Verification items for the finished model (mm, model axes). A direction names the side the tool comes from. Give positions to 0.01 mm unless a question says otherwise; leave off trailing zeros. Write each loop counter-clockwise with the first axis right and the second up, starting at its lowest first coordinate (ties: lowest second). Pieces come first, ordered by that corner, then holes. Notation, with made-up numbers: (67.5, 51.5) -> (124.5, 51.5) arc R11 ccw to (124.5, 56.5) -> close; hole circle Ø10 at (37.25, 61). An arc over 180 degrees is marked (long way). Answer as CSV lines item,"result".
Autodesk Inventor part; units mm, degrees
ref_plane "YZ Plane" through (0, 0, 0) normal (1, 0, 0) x (0, 1, 0)
ref_plane "XZ Plane" through (0, 0, 0) normal (0, 1, 0) x (-1, 0, 0)
ref_plane "XY Plane" through (0, 0, 0) normal (0, 0, 1) x (1, 0, 0)
sketch "Sketch1" plane through (0, 0, 0) normal (0, 1, 0) x (-1, 0, 0)
  circle A0 centre (-31.5089, -30.9076) radius 2.1844
  circle A1 centre (-31.5089, 40.6188) radius 2.1844
  circle A2 centre (44.6911, -30.9076) radius 2.1844
  circle A3 centre (44.6911, 40.6188) radius 2.1844
  circle A4 centre (44.6911, 40.6188) radius 6.35
  circle A5 centre (44.6911, -30.9076) radius 6.35
  circle A6 centre (-31.5089, -30.9076) radius 6.35
  circle A7 centre (-31.5089, 40.6188) radius 6.35
  line L0 (44.6911, 46.9688) -> (-31.5089, 46.9688)
  line L1 (-37.8589, 40.6188) -> (-37.8589, -30.9076)
  line L2 (-31.5089, -37.2576) -> (44.6911, -37.2576)
  line L3 (51.0411, -30.9076) -> (51.0411, 40.6188)
  line L4 (44.6911, 34.2688) -> (-31.5089, 34.2688)
  line L5 (-25.1589, 40.6188) -> (-25.1589, -30.9076)
  line L6 (-31.5089, -24.5576) -> (44.6911, -24.5576)
  line L7 (38.3411, 40.6188) -> (38.3411, -30.9076)
  line L8 (38.3411, 35.5878) -> (38.3411, 29.2378)
  line L9 (-25.1589, -24.5576) -> (-25.1589, -18.2076)
  line L10 (-25.1589, 34.2688) -> (-25.1589, 27.9188)
  line L11 (38.3411, -24.5576) -> (38.3411, -21.3826)
  line L12 (38.3411, -24.5576) -> (35.1661, -24.5576)
  line L13 (38.3411, 34.2688) -> (38.3411, 27.9188)
  line L14 (38.3411, -24.5576) -> (31.9911, -24.5576)
  circle A8 centre (-31.5089, 40.6188) radius 3.175
  circle A9 centre (44.6911, 40.6188) radius 3.175
  circle A10 centre (44.6911, -30.9076) radius 3.175
  circle A11 centre (-31.5089, -30.9076) radius 3.175
  line L15 (42.5182, 42.9337) -> (-33.6818, -28.5927)
  line L16 (46.8641, 38.3039) -> (-29.3359, -33.2225)
  line L17 (-29.3359, 42.9337) -> (46.8641, -28.5927)
  line L18 (-33.6818, 38.3039) -> (42.5182, -33.2225)
  arc A12 (31.6495, 32.7316) -> (31.041, 34.2688) centre (31.041, 33.3798) ccw
  arc A13 (38.3411, 28.2499) -> (36.8437, 28.8981) centre (37.4521, 28.2499) ccw
  arc A14 (36.8437, -19.1869) -> (38.3411, -18.5387) centre (37.4521, -18.5387) ccw
  arc A15 (31.041, -24.5576) -> (31.6495, -23.0204) centre (31.041, -23.6686) ccw
  arc A16 (-17.8588, 34.2688) -> (-18.4672, 32.7316) centre (-17.8588, 33.3798) ccw
  arc A17 (-23.6614, 28.8981) -> (-25.1589, 28.2499) centre (-24.2699, 28.2499) ccw
  arc A18 (-25.1589, -18.5387) -> (-23.6614, -19.1869) centre (-24.2699, -18.5387) ccw
  arc A19 (-18.4672, -23.0204) -> (-17.8588, -24.5576) centre (-17.8588, -23.6686) ccw
  point P0 (-25.1589, 30.3037)
  point P1 (1.952, 4.8556)
  point P2 (-25.1589, -20.5925)
  point P3 (-20.1048, 34.2688)
  point P4 (33.2871, 34.2688)
  point P5 (6.5911, 9.2102)
  point P6 (6.5911, 0.501)
  point P7 (-20.1048, -24.5576)
  point P8 (11.2303, 4.8556)
  point P9 (-25.1589, 28.2499)
  point P10 (-25.1589, -18.5387)
  dimension "d0" = 12.7
  dimension "d1" = 12.7
  dimension "d2" = 12.7
  dimension "d3" = 12.7
  dimension "d8" = 6.35
  dimension "d11" = 6.35
  dimension "d14" = 6.35
  dimension "d16" = 6.35
  dimension "d17" = 6.35
  dimension "d18" = 6.35
  dimension "d19" = 6.35
  dimension "d20" = 6.35
  dimension "d21" = 0.889
  dimension "d22" = 0.889
  dimension "d23" = 0.889
  dimension "d24" = 0.889
  dimension "d25" = 0.889
  dimension "d26" = 0.889
  dimension "d27" = 0.889
  dimension "d28" = 0.889
extrude "Extrusion1" add sketch "Sketch1" along normal blind 1.5875 contours A4 L16 A9 L15 | L3 A5 L6 L17 L7 L16 L4 A4 | A4 L7 L15 L4 L17 L5 A7 L0 | L4 L16 A4 | A5 L18 A10 L17 | A4 L15 L7 | A7 L17 A8 L18 | L16 L4 L7 L15 A4 | A4 L15 A9 L16 | L16 L7 L4 | A5 L17 L6 | L2 A6 L5 L16 L6 L18 L7 A5 | L7 L4 L15 | L5 L17 A7 | A7 L4 L18 L5 L15 L6 A6 L1 | A9 | L7 L16 L17 L15 L4 | L7 A13 L16 | L17 A10 L18 A5 | A5 L18 L7 L6 L17 | L6 L7 L17 | L7 L18 A5 | A6 L15 A11 L16 | L15 A12 L4 | L17 L5 L4 L18 A7 | A7 L18 A8 L17 | L17 L4 L5 | A7 L18 L4 | A10 | L7 L18 L6 | L6 L18 L16 L17 L7 | L17 A14 L7 | A6 L16 L5 | A8 | L5 L18 L4 | L4 L17 L15 L18 L5 | L4 A16 L17 | L6 L15 A6 | L16 L18 L15 L17 | L6 A15 L18 | L16 A11 L15 A6 | A6 L15 L6 L5 L16 | L5 L6 L16 | L18 A17 L5 | L15 L5 L6 | L16 L6 L5 L15 L18 | A11 | L16 A19 L6 | L5 A18 L15
properties part number "Hookcrossbrace"
1) Tool access check on faces 1 (the flat face through (10.68, 0.78, -7)), 2 (the flat face through (-6, 0, 5)). Record the directions out of +Z, -Z, +X, -X, +Y, -Y that give a thin tool (end or side, any length) a straight path to the whole face; none if there is none.
Reported:
face 1,"+Y, -Y"
face 2,"+Z, -Z, +X, -X, -Y"
2) Section check C-C (z = 6). Record the boundary of the cut face in (x, y).
Reported:
outline,"(-51.04, 0) -> (-38.34, 0) -> (-38.34, 1.59) -> (-51.04, 1.59) -> close; (-12.45, 0) -> (-0.73, 0) -> (-0.73, 1.59) -> (-12.45, 1.59) -> close; (25.16, 0) -> (37.86, 0) -> (37.86, 1.59) -> (25.16, 1.59) -> close"
3) Section check A-A (y = 1.1). State how many separate pieces and enclosed holes the cut face has, and give its area (3 significant figures).
Reported:
separate pieces,"1"
enclosed holes,"8"
area,"4,680 mm²"
4) Section check D-D (x = -13). Record the boundary of the cut face in (y, z).
Reported:
outline,"(0, -37.26) -> (1.59, -37.26) -> (1.59, -24.56) -> (0, -24.56) -> close; (0, -5.51) -> (1.59, -5.51) -> (1.59, 3.19) -> (0, 3.19) -> close; (0, 6.52) -> (1.59, 6.52) -> (1.59, 15.23) -> (0, 15.23) -> close; (0, 34.27) -> (1.59, 34.27) -> (1.59, 46.97) -> (0, 46.97) -> close"
5) Section check B-B (x = -3). Record the boundary of the cut face in (y, z).
Reported:
outline,"(0, -37.26) -> (1.59, -37.26) -> (1.59, -24.56) -> (0, -24.56) -> close; (0, -2.87) -> (1.59, -2.87) -> (1.59, 12.58) -> (0, 12.58) -> close; (0, 34.27) -> (1.59, 34.27) -> (1.59, 46.97) -> (0, 46.97) -> close"
6) Scan lines: line 1 along Z through (x, y) = (0.5, 0.1); line 2 along X through (y, z) = (1.3, 19); line 3 along X through (y, z) = (1, -6). Record each from-to range of solid material in increasing order.
Reported:
line 1,"-37.26 to -24.56, -6.16 to 2.55, 7.16 to 15.87, 34.27 to 46.97"
line 2,"-51.04 to -38.34, -26.3 to -17.02, 3.84 to 13.12, 25.16 to 37.86"
line 3,"-51.04 to -38.34, -22.8 to -13.52, 0.33 to 9.61, 25.16 to 37.86"
7) Draft check along Z on faces 3 (the cylindrical face through (35.949, 0.783, -35.447)), 4 (the flat face through (-6, 1.588, 5)), 5 (the flat face through (5.763, 0.783, -11.095)), 6 (the cylindrical face through (-45.9, 0.8, 38.8)). Enter one of: +Z half, -Z half, draft (parallel to the pull), parting line (faces both ways), or undercut.
Reported:
face 3,"-Z half"
face 4,"draft"
face 5,"undercut"
face 6,"undercut"
